from build123d import *

# Parameters (mm, degrees)
SKETCH1_R           = 19.5
BOSS_EXTRUDE1_DEPTH = 2
SKETCH2_R           = 4.5
BOSS_EXTRUDE2_DEPTH = 8
SKETCH3_R           = 4.5
BOSS_EXTRUDE3_DEPTH = 1
SKETCH4_R           = 2
CUT_EXTRUDE1_DEPTH  = 11
CUT_EXTRUDE5_DEPTH  = 2
CIRPATTERN1_COUNT   = 56


with BuildPart() as part:
    # Sketch1 → Boss-Extrude1 (new body)
    with BuildSketch(Plane(origin=(0, 0, 0), x_dir=(0, 0, -1), z_dir=(1, 0, 0))):
        Circle(SKETCH1_R)
    extrude(amount=BOSS_EXTRUDE1_DEPTH)

    # Sketch2 → Boss-Extrude2 (add)
    with BuildSketch(Plane(origin=(2, 0, 0), x_dir=(0, 0, -1), z_dir=(1, 0, 0))):
        Circle(SKETCH2_R)
    extrude(amount=BOSS_EXTRUDE2_DEPTH)

    # Sketch3 → Boss-Extrude3 (add)
    with BuildSketch(Plane.ZY):
        Circle(SKETCH3_R)
    extrude(amount=BOSS_EXTRUDE3_DEPTH)

    # Sketch4 → Cut-Extrude1 (cut)
    with BuildSketch(Plane(origin=(10, 0, 0), x_dir=(0, 0, -1), z_dir=(1, 0, 0))):
        Circle(SKETCH4_R)
    extrude(amount=-CUT_EXTRUDE1_DEPTH, mode=Mode.SUBTRACT)

    # Sketch5 → Cut-Extrude5 (cut)
    with BuildSketch(Plane.ZY):
        with BuildLine():
            Line((-1.093373721, 19.469322893), (0, 18))
            Line((0, 18), (1.09337372, 19.469322893))
            ThreePointArc((1.09337372, 19.469322893), (-1e-09, 19.5), (-1.093373721, 19.469322893))
        make_face()
    cut_extrude5 = extrude(amount=-CUT_EXTRUDE5_DEPTH, mode=Mode.SUBTRACT)

    # CirPattern1: Cut-Extrude5 ×56 about axis
    cirpattern1_axis = Axis((0, 0, 0), (1, 0, 0))
    for i in range(1, CIRPATTERN1_COUNT):
        add(cut_extrude5.rotate(cirpattern1_axis, i * 360 / CIRPATTERN1_COUNT), mode=Mode.SUBTRACT)


solid = part.part
Read the model definition and answer for the solid it produces. Units are mm, in the model's axes. A direction names the side the tool comes from. Coordinates: 2 decimals unless noted, no trailing zeros. Loops run counter-clockwise (first coordinate to the right, second up) from the corner with the lowest first, then second, coordinate; pieces in that order, holes last.
Q1. Which of the six approach directions +Z, -Z, +X, -X, +Y, -Y give full straight-line access (tool end or side, diameter ignored) to faces 1 (the face through (0.986, -18.689, -1.548)), 2 (the face through (1, -6.7, -17.5)), 3 (the face through (0.986, 17.129, 7.634))?
Q2. Each of these flat-tipped pins is pushed along its axis until it touches: pin 1 Ø12 at (y, z) = (8.5, 8) entering from +X; pin 2 Ø1.5 at (x, z) = (4.5, 9) entering from -Y; pin 3 Ø1 at (y, z) = (6, 1.5) entering from -X; pin 4 Ø5 at (x, z) = (0, 14.5) entering from +Y. Where does it stop, or does it pass through?
Q3. Consider probe 1 along Y at (x, z) = (2.75, 0); probe 2 along X at (y, z) = (2.5, -16.5); probe 3 along Y at (x, z) = (-0.5, -1). Determine where each line is inside the solid, lowest interval first.
Q4. The part is cut by section B-B on y = 2.5. Write down the section's boundary in (x, z), and give its area (3 significant figures).
Q5. The part is cut by section C-C on z = -12. Write down the section's boundary in (x, y).
Q6. The part is cut by section A-A on x = 5.5. Write down the section's boundary in (y, z), and give its area (3 significant figures).
Results below:
1. face 1: +X, -X, -Y
1. face 2: -Z, +X, -X
1. face 3: +X, -X, +Y
2. pin 1: stops at x = 2
2. pin 2: passes through
2. pin 3: stops at x = 0
2. pin 4: stops at y = 14.54
3. probe 1: y = -4.5 to -2, 2 to 4.5
3. probe 2: x = 0 to 2
3. probe 3: y = -4.39 to -1.73, 1.73 to 4.39
4. outline: (-1, -3.74) - (0, -3.74) - (0, -18.41) - (2, -18.41) - (2, -3.74) - (10, -3.74) - (10, 3.74) - (2, 3.74) - (2, 18.41) - (0, 18.41) - (0, 3.74) - (-1, 3.74) - close
4. area: 141 mm2
5. outline: (0, -14.28) - (2, -14.28) - (2, 14.28) - (0, 14.28) - close
6. outline: circle Ø9 at (0, 0); hole circle Ø4 at (0, 0)
6. area: 51.1 mm2
